Model file for the job. Use its own axes, mm. Coordinates: 2 decimals unless noted, no trailing zeros. Loops run counter-clockwise (first coordinate to the right, second up) from the corner with the lowest first, then second, coordinate; pieces in that order, holes last.
Autodesk Inventor part; units mm, degrees
ref_plane "YZ Plane" through (0, 0, 0) normal (1, 0, 0) x (0, 1, 0)
ref_plane "XZ Plane" through (0, 0, 0) normal (0, 1, 0) x (-1, 0, 0)
ref_plane "XY Plane" through (0, 0, 0) normal (0, 0, 1) x (1, 0, 0)
sketch "Sketch1" plane through (0, 0, 0) normal (1, 0, 0) x (0, 1, 0)
  line L0 (25.0568, 85.4307) -> (-25.9432, 85.4307)
  line L1 (-25.9432, 85.4307) -> (-25.9432, -79.5693)
  line L2 (-25.9432, -79.5693) -> (25.0568, -79.5693)
  line L3 (25.0568, -79.5693) -> (25.0568, 85.4307)
  point P0 (0, 0)
  dimension "d0" = 165
  dimension "d1" = 51
extrude "Extrusion1" add sketch "Sketch1" along normal blind 3
fillet "Fillet1" radius 3 4 edges at (1.5, 25.0568, 85.4307) (1.5, -25.9432, 85.4307) (1.5, 25.0568, -79.5693) (1.5, -25.9432, -79.5693)
sketch "Sketch2" plane through (3, 0, 0) normal (1, 0, 0) x (0, 0, -1)
  line L0 (-77.4307, 22.0568) -> (71.5693, 22.0568)
  line L1 (71.5693, 22.0568) -> (71.5693, -22.9432)
  line L2 (71.5693, -22.9432) -> (-77.4307, -22.9432)
  line L3 (-77.4307, -22.9432) -> (-77.4307, 22.0568)
  line L4 (-85.4307, 22.0568) -> (-85.4307, -22.9432)
  line L5 (79.5693, -22.9432) -> (79.5693, 22.0568)
  line L6 (-82.4307, -25.9432) -> (76.5693, -25.9432)
  line L7 (76.5693, 25.0568) -> (-82.4307, 25.0568)
  point P0 (0, 0)
  dimension "d5" = 149
  dimension "d6" = 45
  dimension "d9" = 165
  dimension "d10" = 8
  dimension "d11" = 51
  dimension "d12" = 3
extrude "Extrusion2" cut sketch "Sketch2" against normal blind 0.1
sketch "Sketch4" plane through (2.9, 0, 0) normal (1, 0, 0) x (0, 0, -1)
  line L0 (-77.4307, 22.0568) -> (71.5693, 22.0568)
  line L1 (71.5693, 22.0568) -> (71.5693, -22.9432)
  line L2 (71.5693, -22.9432) -> (-77.4307, -22.9432)
  line L3 (-77.4307, -22.9432) -> (-77.4307, 22.0568)
  line L4 (-41.5807, 1.8676) -> (-33.2807, 1.8676)
  line L5 (-33.2807, 1.8676) -> (-33.2807, -2.7541)
  line L6 (-33.2807, -2.7541) -> (-41.5807, -2.7541)
  line L7 (-41.5807, -2.7541) -> (-41.5807, 1.8676)
  line L8 (-41.5807, 1.8676) -> (-33.2807, -2.7541) construction
  line L9 (-33.2807, 1.8676) -> (-41.5807, -2.7541) construction
  arc A0 (-33.2807, 1.8676) -> (-41.5807, 1.8676) centre (-37.4307, -0.4432) ccw
  line L10 (-12.5807, 6.7459) -> (-4.2807, 6.7459)
  line L11 (-4.2807, 6.7459) -> (-4.2807, 11.3676)
  line L12 (-4.2807, 11.3676) -> (-12.5807, 11.3676)
  line L13 (-12.5807, 11.3676) -> (-12.5807, 6.7459)
  line L14 (-12.5807, 6.7459) -> (-4.2807, 11.3676) construction
  line L15 (-4.2807, 6.7459) -> (-12.5807, 11.3676) construction
  arc A1 (-4.2807, 11.3676) -> (-12.5807, 11.3676) centre (-8.4307, 9.0568) ccw
  arc A2 (-12.5807, 6.7459) -> (-4.2807, 6.7459) centre (-8.4307, 9.0568) ccw
  line L16 (7.4193, 11.3676) -> (15.7193, 11.3676)
  line L17 (15.7193, 11.3676) -> (15.7193, 6.7459)
  line L18 (15.7193, 6.7459) -> (7.4193, 6.7459)
  line L19 (7.4193, 6.7459) -> (7.4193, 11.3676)
  line L20 (7.4193, 11.3676) -> (15.7193, 6.7459) construction
  line L21 (15.7193, 11.3676) -> (7.4193, 6.7459) construction
  arc A3 (15.7193, 11.3676) -> (7.4193, 11.3676) centre (11.5693, 9.0568) ccw
  arc A4 (7.4193, 6.7459) -> (15.7193, 6.7459) centre (11.5693, 9.0568) ccw
  line L22 (27.4193, 6.7459) -> (35.7193, 6.7459)
  line L23 (35.7193, 6.7459) -> (35.7193, 11.3676)
  line L24 (35.7193, 11.3676) -> (27.4193, 11.3676)
  line L25 (27.4193, 11.3676) -> (27.4193, 6.7459)
  line L26 (27.4193, 6.7459) -> (35.7193, 11.3676) construction
  line L27 (35.7193, 6.7459) -> (27.4193, 11.3676) construction
  line L28 (55.7193, -12.2541) -> (47.4193, -12.2541)
  line L29 (47.4193, -12.2541) -> (47.4193, -7.6324)
  line L30 (47.4193, -7.6324) -> (55.7193, -7.6324)
  line L31 (55.7193, -7.6324) -> (55.7193, -12.2541)
  line L32 (55.7193, -12.2541) -> (47.4193, -7.6324) construction
  line L33 (47.4193, -12.2541) -> (55.7193, -7.6324) construction
  line L34 (27.4193, -12.2541) -> (35.7193, -12.2541)
  line L35 (35.7193, -12.2541) -> (35.7193, -7.6324)
  line L36 (35.7193, -7.6324) -> (27.4193, -7.6324)
  line L37 (27.4193, -7.6324) -> (27.4193, -12.2541)
  line L38 (27.4193, -12.2541) -> (35.7193, -7.6324) construction
  line L39 (35.7193, -12.2541) -> (27.4193, -7.6324) construction
  line L40 (15.7193, -12.2541) -> (7.4193, -12.2541)
  line L41 (7.4193, -12.2541) -> (7.4193, -7.6324)
  line L42 (7.4193, -7.6324) -> (15.7193, -7.6324)
  line L43 (15.7193, -7.6324) -> (15.7193, -12.2541)
  line L44 (15.7193, -12.2541) -> (7.4193, -7.6324) construction
  line L45 (7.4193, -12.2541) -> (15.7193, -7.6324) construction
  line L46 (-12.5807, -12.2541) -> (-4.2807, -12.2541)
  line L47 (-4.2807, -12.2541) -> (-4.2807, -7.6324)
  line L48 (-4.2807, -7.6324) -> (-12.5807, -7.6324)
  line L49 (-12.5807, -7.6324) -> (-12.5807, -12.2541)
  line L50 (-12.5807, -12.2541) -> (-4.2807, -7.6324) construction
  line L51 (-4.2807, -12.2541) -> (-12.5807, -7.6324) construction
  arc A5 (-4.2807, -7.6324) -> (-12.5807, -7.6324) centre (-8.4307, -9.9432) ccw
  arc A6 (-12.5807, -12.2541) -> (-4.2807, -12.2541) centre (-8.4307, -9.9432) ccw
  arc A7 (15.7193, -7.6324) -> (7.4193, -7.6324) centre (11.5693, -9.9432) ccw
  arc A8 (7.4193, -12.2541) -> (15.7193, -12.2541) centre (11.5693, -9.9432) ccw
  arc A9 (35.7193, -7.6324) -> (27.4193, -7.6324) centre (31.5693, -9.9432) ccw
  arc A10 (27.4193, -12.2541) -> (35.7193, -12.2541) centre (31.5693, -9.9432) ccw
  arc A11 (55.7193, -7.6324) -> (47.4193, -7.6324) centre (51.5693, -9.9432) ccw
  arc A12 (47.4193, -12.2541) -> (55.7193, -12.2541) centre (51.5693, -9.9432) ccw
  arc A13 (35.7193, 11.3676) -> (27.4193, 11.3676) centre (31.5693, 9.0568) ccw
  arc A14 (27.4193, 6.7459) -> (35.7193, 6.7459) centre (31.5693, 9.0568) ccw
  line L52 (55.7193, 6.7459) -> (47.4193, 6.7459)
  line L53 (47.4193, 6.7459) -> (47.4193, 11.3676)
  line L54 (47.4193, 11.3676) -> (55.7193, 11.3676)
  line L55 (55.7193, 11.3676) -> (55.7193, 6.7459)
  line L56 (55.7193, 6.7459) -> (47.4193, 11.3676) construction
  line L57 (47.4193, 6.7459) -> (55.7193, 11.3676) construction
  arc A15 (55.7193, 11.3676) -> (47.4193, 11.3676) centre (51.5693, 9.0568) ccw
  arc A16 (47.4193, 6.7459) -> (55.7193, 6.7459) centre (51.5693, 9.0568) ccw
  arc A17 (-41.5807, -2.7541) -> (-33.2807, -2.7541) centre (-37.4307, -0.4432) ccw
  line L58 (-70.4307, -8.4432) -> (-70.4307, 7.5568)
  line L59 (-70.4307, 7.5568) -> (-54.4307, 7.5568)
  line L60 (-54.4307, 7.5568) -> (-54.4307, -8.4432)
  line L61 (-54.4307, -8.4432) -> (-70.4307, -8.4432)
  line L62 (-70.4307, -8.4432) -> (-54.4307, 7.5568) construction
  line L63 (-70.4307, 7.5568) -> (-54.4307, -8.4432) construction
  point P0 (0, 0)
  point P1 (-62.4307, -0.4432)
  point P2 (-62.4307, -13.1432)
  point P3 (-62.4307, 12.2568)
  dimension "d16" = 20
  dimension "d17" = 20
  dimension "d18" = 20
  dimension "d20" = 19
  dimension "d25" = 20
  dimension "d26" = 20
  dimension "d27" = 20
  dimension "d28" = 19
  dimension "d29" = 19
  dimension "d43" = 13
  dimension "d44" = 45
  dimension "d45" = 13
  dimension "d46" = 13
  dimension "d47" = 13
  dimension "d70" = 22.5
  dimension "d71" = 8.3
  dimension "d72" = 4.75
  dimension "d73" = 40
  dimension "d74" = 20.1892
  dimension "d75" = 8.3
  dimension "d76" = 4.75
  dimension "d77" = 8.3
  dimension "d78" = 4.75
  dimension "d79" = 8.3
  dimension "d81" = 8.3
  dimension "d82" = 8.3
  dimension "d83" = 8.3
  dimension "d84" = 8.3
  dimension "d85" = 4.75
  dimension "d86" = 4.75
  dimension "d88" = 4.75
  dimension "d90" = 4.75
  dimension "d98" = 20
  dimension "d100" = 20
  dimension "d101" = 8.3
  dimension "d104" = 16
  dimension "d105" = 16
  dimension "d106" = 15
  dimension "d107" = 22.5
  dimension "d108" = 8
  dimension "d109" = 8
  dimension "d110" = 12.7
  dimension "d111" = 12.7
extrude "Extrusion3" cut sketch "Sketch4" against normal blind 20 contours A0 L4 | L4 L5 L6 L7 | L6 A17 | L13 L12 L11 L10 | L10 A2 | A1 L12 | A3 L16 | L16 L17 L18 L19 | L18 A4 | L25 L24 L23 L22 | L22 A14 | A13 L24 | A12 L28 | L28 L29 L30 L31 | L30 A11 | L37 L36 L35 L34 | L34 A10 | A9 L36 | A8 L40 | L40 L41 L42 L43 | L42 A7 | L49 L48 L47 L46 | L46 A6 | A5 L48 | A16 L52 | L52 L53 L54 L55 | L54 A15 | L58 L59 L60 L61
fillet "Fillet2" radius 1 4 edges at (1.45, 7.5568, 54.4307) (1.45, -8.4432, 54.4307) (1.45, -8.4432, 70.4307) (1.45, 7.5568, 70.4307)
hole "Hole4" at (2.9, -0.4432, 37.4307) at (2.9, 9.0568, -11.5693) at (2.9, 9.0568, 8.4307) at (2.9, 9.0568, -31.5693) at (2.9, 9.0568, -51.5693) at (2.9, -9.9432, 8.4307) at (2.9, -9.9432, -11.5693) at (2.9, -9.9432, -31.5693) at (2.9, -9.9432, -51.5693) at (2.9, -13.1432, 62.4307) at (2.9, 12.2568, 62.4307) direction (-1, 0, 0) diameter 3.4 end through all
sketch "Sketch9" plane through (3, 0, 0) normal (1, 0, 0) x (0, 0, -1)
  line L0 (-77.4307, -22.9432) -> (-77.4307, 22.0568)
  line L1 (-77.4307, 22.0568) -> (71.5693, 22.0568)
  line L2 (71.5693, 22.0568) -> (71.5693, -22.9432)
  line L3 (71.5693, -22.9432) -> (-77.4307, -22.9432)
  arc A0 (76.5693, -25.9432) -> (79.5693, -22.9432) centre (76.5693, -22.9432) ccw
  line L4 (79.5693, -22.9432) -> (79.5693, 22.0568)
  arc A1 (79.5693, 22.0568) -> (76.5693, 25.0568) centre (76.5693, 22.0568) ccw
  line L5 (76.5693, 25.0568) -> (-82.4307, 25.0568)
  arc A2 (-82.4307, 25.0568) -> (-85.4307, 22.0568) centre (-82.4307, 22.0568) ccw
  line L6 (-85.4307, 22.0568) -> (-85.4307, -22.9432)
  arc A3 (-85.4307, -22.9432) -> (-82.4307, -25.9432) centre (-82.4307, -22.9432) ccw
  line L7 (-82.4307, -25.9432) -> (76.5693, -25.9432)
  point P0 (0, 0)
extrude "Extrusion4" cut sketch "Sketch9" against normal blind 0.1
equation "\"d10\" = -0.5 * d5 + 0.5 * d9"
equation "\"d12\" = -0.5 * d6 + 0.5 * d11"
equation "\"d78\" = d76"
equation "\"d85\" = d76"
equation "\"d86\" = d85"
equation "\"d88\" = d86"
equation "\"d90\" = d78"
properties part number "Front-panel"
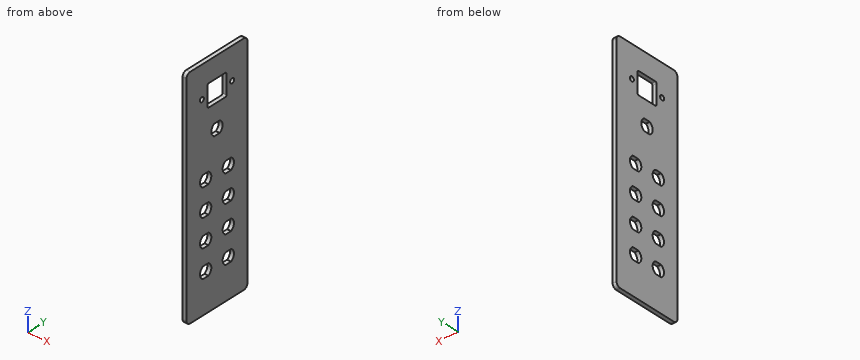
Q1. Slice it at A-A (y = 0). List the corners of the cut face in (x, z), and give its area (3 significant figures).
Answers:
outline: (0, -79.57) - (2.9, -79.57) - (2.9, 33.28) - (0, 33.28) - close; (0, 41.58) - (2.9, 41.58) - (2.9, 54.43) - (0, 54.43) - close; (0, 70.43) - (2.9, 70.43) - (2.9, 85.43) - (0, 85.43) - close
area: 408 mm2
Q2. Slice it at D-D (x = 2.2). Count the separate pieces of the cut face and the enclosed holes in it, and give its area (3 significant figures).
Answers:
separate pieces: 1
enclosed holes: 12
area: 7,530 mm2
Q3. Flat gauge pin, fed straight in: P1, Ø5.5, axis at y = -13.14, z = 62.43, coming from the +X side. Where does the tip first touch, or does it go through?
Answers:
P1: stops at x = 2.9
Q4. Slice it at C-C (z = -32.5). List the corners of the cut face in (x, y).
Answers:
outline: (0, -25.94) - (2.9, -25.94) - (2.9, -14.6) - (0, -14.6) - close; (0, -5.29) - (2.9, -5.29) - (2.9, 4.4) - (0, 4.4) - close; (0, 13.71) - (2.9, 13.71) - (2.9, 25.06) - (0, 25.06) - close
Q5. Drill centre lines: line 1 (Z direction, x = 1.2, y = 10.5); line 2 (Z direction, x = 0.5, y = -1.5); line 3 (Y direction, x = 1.75, z = -52). Where is each one in solid material? Low to high.
Answers:
line 1: z = -79.57 to -55.72, -47.42 to -35.72, -27.42 to -15.72, -7.42 to 4.28, 12.58 to 85.43
line 2: z = -79.57 to 33.28, 41.58 to 54.43, 70.43 to 85.43
line 3: y = -25.94 to -14.67, -5.21 to 4.33, 13.79 to 25.06
Q6. Slice it at B-B (z = 57). List the corners of the cut face in (x, y), and give its area (4 significant figures).
Answers:
outline: (0, -25.94) - (2.9, -25.94) - (2.9, -8.44) - (0, -8.44) - close; (0, 7.56) - (2.9, 7.56) - (2.9, 25.06) - (0, 25.06) - close
area: 101.5 mm2
